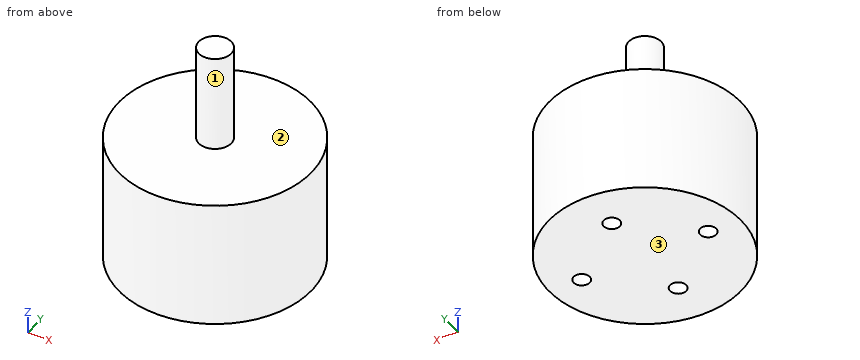
```python
from build123d import *

# Parameters (mm, degrees)
SKETCH1_R           = 14.351
BOSS_EXTRUDE1_DEPTH = 19.05
SKETCH2_R           = 2.4257
BOSS_EXTRUDE2_DEPTH = 14.478
SKETCH3_R           = 1.2065
CUT_EXTRUDE1_DEPTH  = 5.08


with BuildPart() as part:
    # Sketch1 → Boss-Extrude1 (new body)
    with BuildSketch(Plane.XY):
        with Locations(Location((0, 0, 0), (0, 0, 180))):
            Circle(SKETCH1_R)
    extrude(amount=BOSS_EXTRUDE1_DEPTH)

    # Sketch2 → Boss-Extrude2 (add)
    with BuildSketch(Plane.XY.offset(19.05)):
        Circle(SKETCH2_R)
    extrude(amount=BOSS_EXTRUDE2_DEPTH)

    # Sketch3 → Cut-Extrude1 (cut)
    with BuildSketch(Plane(origin=(0, 0, 0), x_dir=(-1, 0, 0), z_dir=(0, 0, -1))):
        with Locations((0, 8.001)):
            Circle(SKETCH3_R)
        with Locations((9.525, 0)):
            Circle(SKETCH3_R)
        with Locations((0, -8.001)):
            Circle(SKETCH3_R)
        with Locations((-9.525, 0)):
            Circle(SKETCH3_R)
    extrude(amount=-CUT_EXTRUDE1_DEPTH, mode=Mode.SUBTRACT)


solid = part.part
```
The model under review builds one solid part; all positions refer to its coordinate system, in mm. Face numbers are marked on the shaded views. Give positions to 0.01 mm unless a question says otherwise; leave off trailing zeros. Write each loop counter-clockwise with the first axis right and the second up, starting at its lowest first coordinate (ties: lowest second). Pieces come first, ordered by that corner, then holes. Notation, with made-up numbers: M 74.25,60 L 103.25,60 A28 ccw 103.25,99 Z; hole C -28,-12.5 d6. An arc over 180 degrees is marked long. Answer in a Markdown table with one row per item.
Item 1: For P1, Ø1, axis at x = -0.5, y = -8, coming from the +Z side; P2, Ø6, axis at y = 10, z = 11.5, coming from the +X side; P3, Ø0.7, axis at x = -9.5, y = 0, coming from the -Z side, all flat-tipped, find the tip position at first contact; note any pin that passes through.
Check sheet entries:
| item | result |
|---|---|
| P1 | z = 19.05 |
| P2 | x = 12.53 |
| P3 | z = 5.08 |
Item 2: Draft analysis for pull direction Z (two halves, no side actions). For the marked faces 1, 2 and 3, state which applies: +Z half, -Z half, draft (parallel to the pull), parting line (faces both ways), or undercut.
Check sheet entries:
| item | result |
|---|---|
| face 1 | draft |
| face 2 | +Z half |
| face 3 | -Z half |
Item 3: For line 1 along Y through (x, z) = (0, 1.2); line 2 along Z through (x, y) = (-11.75, -0.5); line 3 along Y through (x, z) = (11, 2), list the stretches that pass through material, from the lowest coordinate up.
Check sheet entries:
| item | result |
|---|---|
| line 1 | -14.35 to -9.21, -6.79 to 6.79, 9.21 to 14.35 |
| line 2 | 0 to 19.05 |
| line 3 | -9.22 to 9.22 |
Item 4: Add section B-B on y = 0. Give the boundary of the cut face in (x, z).
Check sheet entries:
| item | result |
|---|---|
| outline | M -14.35,0 L -10.73,0 L -10.73,5.08 L -8.32,5.08 L -8.32,0 L 8.32,0 L 8.32,5.08 L 10.73,5.08 L 10.73,0 L 14.35,0 L 14.35,19.05 L 2.43,19.05 L 2.43,33.53 L -2.43,33.53 L -2.43,19.05 L -14.35,19.05 Z |
Item 5: Add section D-D on z = 25. Give the boundary of the cut face in (x, y).
Check sheet entries:
| item | result |
|---|---|
| outline | C 0,0 d4.85 |
Item 6: Add section A-A on x = 0. Give the boundary of the cut face in (y, z).
Check sheet entries:
| item | result |
|---|---|
| outline | M -14.35,0 L -9.21,0 L -9.21,5.08 L -6.79,5.08 L -6.79,0 L 6.79,0 L 6.79,5.08 L 9.21,5.08 L 9.21,0 L 14.35,0 L 14.35,19.05 L 2.43,19.05 L 2.43,33.53 L -2.43,33.53 L -2.43,19.05 L -14.35,19.05 Z |
Item 7: Add section C-C on z = 12. Give the boundary of the cut face in (x, y), plus the area to 3 significant figures.
Check sheet entries:
| item | result |
|---|---|
| outline | C 0,0 d28.7 |
| area | 647 mm2 |
